The model under review builds one solid part; all positions refer to its coordinate system, in mm. Coordinates: 2 decimals unless noted, no trailing zeros. Order: outer loops, then holes, each group sorted by start corner. A loop starts at its lowest first (then second) coordinate and runs counter-clockwise, first axis right, second up. Notation, with made-up numbers: M -37.75,-4.75 L -27.75,-4.75 A31 cw -27.75,29.25 Z; hole C 20,41 d3. An arc over 180 degrees is marked long. Write each question's results on one line, items separated by ' | '.
Autodesk Inventor part; units mm, degrees
ref_plane "YZ Plane" through (0, 0, 0) normal (1, 0, 0) x (0, 1, 0)
ref_plane "XZ Plane" through (0, 0, 0) normal (0, 1, 0) x (-1, 0, 0)
ref_plane "XY Plane" through (0, 0, 0) normal (0, 0, 1) x (1, 0, 0)
sketch "Sketch1" plane through (0, 0, 0) normal (0, 1, 0) x (-1, 0, 0)
  line L0 (0, 0) -> (0, 215.9)
  line L1 (0, 215.9) -> (304.8, 215.9)
  line L2 (0, 0) -> (774.7, 0)
  line L3 (0, 0) -> (0, -215.9)
  line L4 (0, -215.9) -> (304.8, -215.9)
  line L5 (774.7, 0) -> (774.7, -165.1)
  line L6 (774.7, -165.1) -> (774.7, 0)
  line L7 (774.7, 0) -> (774.7, 165.1)
  line L8 (774.7, 165.1) -> (304.8, 215.9)
  line L9 (774.7, -165.1) -> (304.8, -215.9)
  line L10 (0, -215.9) -> (76.2, -215.9)
  line L11 (76.2, -215.9) -> (76.2, -177.8)
  line L12 (304.8, -215.9) -> (228.6, -215.9)
  line L13 (228.6, -215.9) -> (228.6, -177.8)
  line L14 (774.7, 0) -> (774.7, -101.6)
  line L15 (774.7, -101.6) -> (749.3, -101.6)
  line L16 (774.7, 0) -> (774.7, 101.6)
  line L17 (774.7, 101.6) -> (749.3, 101.6)
  line L18 (0, 215.9) -> (76.2, 215.9)
  line L19 (76.2, 215.9) -> (76.2, 177.8)
  line L20 (304.8, 215.9) -> (228.6, 215.9)
  line L21 (228.6, 215.9) -> (228.6, 177.8)
  line L22 (0, 0) -> (25.4, 0)
  line L23 (774.7, -165.1) -> (597.93, -184.2103)
  line L24 (597.93, -184.2103) -> (593.8349, -146.331)
  line L25 (597.93, -184.2103) -> (421.16, -203.3205)
  line L26 (421.16, -203.3205) -> (417.0649, -165.4413)
  line L27 (774.7, 165.1) -> (597.93, 184.2103)
  line L28 (597.93, 184.2103) -> (593.8349, 146.331)
  line L29 (597.93, 184.2103) -> (421.16, 203.3205)
  line L30 (421.16, 203.3205) -> (417.0649, 165.4413)
  dimension "d0" = 215.9
  dimension "d1" = 304.8
  dimension "d2" = 774.7
  dimension "d3" = 215.9
  dimension "d4" = 304.8
  dimension "d5" = 165.1
  dimension "d6" = 165.1
  dimension "d9" = 76.2
  dimension "d10" = 38.1
  dimension "d11" = 76.2
  dimension "d12" = 38.1
  dimension "d15" = 101.6
  dimension "d16" = 25.4
  dimension "d17" = 101.6
  dimension "d18" = 25.4
  dimension "d23" = 76.2
  dimension "d24" = 38.1
  dimension "d25" = 76.2
  dimension "d26" = 38.1
  dimension "d32" = 25.4
  dimension "d34" = 177.8
  dimension "d35" = 38.1
  dimension "d36" = 177.8
  dimension "d37" = 38.1
  dimension "d38" = 177.8
  dimension "d39" = 38.1
  dimension "d40" = 177.8
  dimension "d41" = 38.1
extrude "Extrusion1" add sketch "Sketch1" along normal blind 3.175
hole "Hole1" at (-593.8349, 0, -146.331) at (-417.0649, 0, -165.4413) at (-228.6, 0, -177.8) at (-76.2, 0, -177.8) at (-76.2, 0, 177.8) at (-228.6, 0, 177.8) at (-417.0649, 0, 165.4413) at (-593.8349, 0, 146.331) at (-749.3, 0, 101.6) at (-749.3, 0, -101.6) at (-25.4, 0, 0) direction (0, 1, 0) diameter 5.1054 end through all
properties part number "frontfloorfit2"
1) Take a section at B-B on x = -569. State the section outline as (y, z) points (3 decimals).
Solutions:
outline: M 0,-187.338 L 3.175,-187.338 L 3.175,187.338 L 0,187.338 Z
2) To check wall thickness, follow line 1 along Z through (x, y) = (-228.6, 1.4); line 2 along Z through (x, y) = (-749.3, 1.95); line 3 along X through (y, z) = (1.1, 101.6). State the ranges of each line that lie inside material, in increasing order.
Solutions:
line 1: -215.9 to -180.35, -175.25 to 175.25, 180.35 to 215.9 | line 2: -167.85 to -104.15, -99.05 to 99.05, 104.15 to 167.85 | line 3: -774.7 to -751.85, -746.75 to 0
3) Take a section at A-A on y = 1.15. Count the separate pieces of the cut face and the enclosed holes in it, plus the area to 3 significant figures.
Solutions:
separate pieces: 1 | enclosed holes: 11 | area: 310,000 mm2
